Source: CAD feature listing. Evaluate the final solid. Frame: model axes, mm. Face numbers are marked on the shaded views. Give positions to 0.01 mm unless a question says otherwise; leave off trailing zeros. Order: outer loops, then holes, each group sorted by start corner. A loop starts at its lowest first (then second) coordinate and runs counter-clockwise, first axis right, second up. Notation, with made-up numbers: M -8,-0.5 L 16,-0.5 A20 cw 16,18.5 Z; hole C -27,20 d10. An arc over 180 degrees is marked long. Answer in a Markdown table with one row per item. Add a question column.
(1) Mould query, pull axis X, two halves, no side actions, for the marked faces 1 and 2. Classes: pulls with the +X half, pulls with the -X half, needs draft (parallel to the pull), parting line crosses it, or undercut.
(2) Material intervals for line 1 along X through (y, z) = (5.7, 0); line 2 along Z through (x, y) = (0, 0.4), sorted ascending.
(3) Section query B-B, the plane x = 0. Return loops of the section in (y, z).
(4) Section query C-C, the plane y = 2.25. Return loops of the section in (x, z), plus the area to 3 significant figures.
(5) Pin query (flat end, axial travel): P1, Ø23.5, axis at x = 1, z = -6, coming from the +Y side; P2, Ø1, axis at y = 2, z = -1.5, coming from the -X side; P3, Ø2, axis at y = 4, z = 15, coming from the +X side; P4, Ø2, axis at y = 4.5, z = 14.5, coming from the -X side. Return the tip coordinate at first contact, or that it passes through.
(6) Section query A-A, the plane z = 0. Return loops of the section in (x, y).
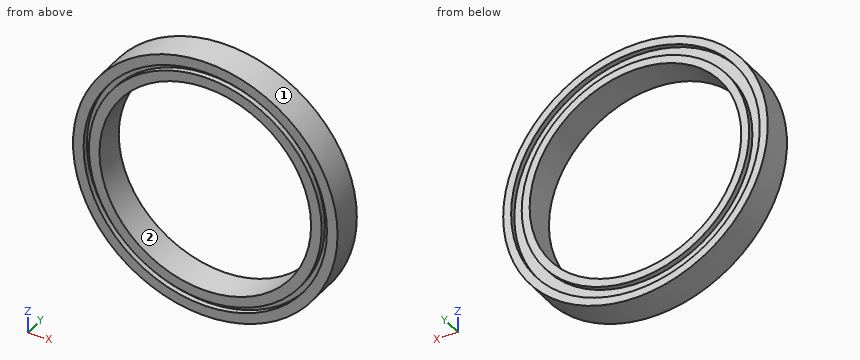
from build123d import *

# Parameters (mm, degrees)
SKETCH1_R           = 25
SKETCH1_R_2         = 20
BOSS_EXTRUDE1_DEPTH = 6
SKETCH2_R           = 23.5
SKETCH2_R_2         = 21.5
CUT_EXTRUDE1_DEPTH  = 1
SKETCH3_R           = 23
SKETCH3_R_2         = 22
CUT_EXTRUDE2_DEPTH  = 1


with BuildPart() as part:
    # Sketch1 → Boss-Extrude1 (new body)
    with BuildSketch(Plane(origin=(0, 0, 0), x_dir=(1, 0, 0), z_dir=(0, 1, 0))):
        Circle(SKETCH1_R)
        Circle(SKETCH1_R_2, mode=Mode.SUBTRACT)
    extrude(amount=BOSS_EXTRUDE1_DEPTH)

    # Sketch2 → Cut-Extrude1 (cut)
    with BuildSketch(Plane(origin=(0, 6, 0), x_dir=(1, 0, 0), z_dir=(0, 1, 0))):
        Circle(SKETCH2_R)
        Circle(SKETCH2_R_2, mode=Mode.SUBTRACT)
    extrude(amount=-CUT_EXTRUDE1_DEPTH, mode=Mode.SUBTRACT)

    # Sketch3 → Cut-Extrude2 (cut)
    with BuildSketch(Plane.XZ):
        Circle(SKETCH3_R)
        Circle(SKETCH3_R_2, mode=Mode.SUBTRACT)
    extrude(amount=-CUT_EXTRUDE2_DEPTH, mode=Mode.SUBTRACT)


solid = part.part
Values follow:
| question | item | result |
|---|---|---|
| 1 | face 1 | parting line crosses it |
| 1 | face 2 | undercut |
| 2 | line 1 | x = -25 to -23.5, -21.5 to -20, 20 to 21.5, 23.5 to 25 |
| 2 | line 2 | z = -25 to -23, -22 to -20, 20 to 22, 23 to 25 |
| 3 | outline | M 0,-25 L 6,-25 L 6,-23.5 L 5,-23.5 L 5,-21.5 L 6,-21.5 L 6,-20 L 0,-20 L 0,-22 L 1,-22 L 1,-23 L 0,-23 Z; M 0,20 L 6,20 L 6,21.5 L 5,21.5 L 5,23.5 L 6,23.5 L 6,25 L 0,25 L 0,23 L 1,23 L 1,22 L 0,22 Z |
| 4 | outline | C 0,0 d50; hole C 0,0 d40 |
| 4 | area | 707 mm² |
| 5 | P1 | passes through |
| 5 | P2 | stops at x = -24.98 |
| 5 | P3 | stops at x = 20.71 |
| 5 | P4 | stops at x = -21.04 |
| 6 | outline | M -25,0 L -23,0 L -23,1 L -22,1 L -22,0 L -20,0 L -20,6 L -21.5,6 L -21.5,5 L -23.5,5 L -23.5,6 L -25,6 Z; M 20,0 L 22,0 L 22,1 L 23,1 L 23,0 L 25,0 L 25,6 L 23.5,6 L 23.5,5 L 21.5,5 L 21.5,6 L 20,6 Z |
